The listing builds one solid part. Answer for the finished solid, in the listing's coordinates (mm). Face numbers are marked on the shaded views. A direction names the side the tool comes from. Give positions to 0.01 mm unless a question says otherwise; leave off trailing zeros. Write each loop counter-clockwise with the first axis right and the second up, starting at its lowest first coordinate (ties: lowest second). Pieces come first, ordered by that corner, then holes. Notation, with made-up numbers: (-19.5, -9.5) -> (15.5, -9.5) arc R21 cw to (15.5, 19.5) -> close; hole circle Ø8 at (-30, 19). An arc over 180 degrees is marked (long way). Use CSV: the item, a comma, the result in double quotes. Start each with the question number.
from build123d import *

# Parameters (mm, degrees)
SKETCH_1_W          = 42
SKETCH_1_H          = 15
EXTRUDE_1_DEPTH     = 5
SKETCH_2_W          = 22
SKETCH_2_H          = 25
EXTRUDE_2_DEPTH     = 9.5
CUT_EXTRUDE_1_DEPTH = 37


with BuildPart() as part:
    # 스케치1 → 보스-돌출1 (new body)
    with BuildSketch(Plane.XY):
        Rectangle(SKETCH_1_W, SKETCH_1_H)
    extrude(amount=EXTRUDE_1_DEPTH)

    # 스케치2 → 보스-돌출2 (add)
    with BuildSketch(Plane.XY.offset(5)):
        Rectangle(SKETCH_2_W, SKETCH_2_H)
    extrude(amount=EXTRUDE_2_DEPTH)

    # 스케치3 → 컷-돌출1 (cut)
    with BuildSketch(Plane(origin=(11, 0, 0), x_dir=(0, 0, -1), z_dir=(1, 0, 0))):
        Polygon((-12.28944968, 12.5), (-5.909253868, -12.5), (-14.5, -12.5), (-14.5, 12.5), align=None)
    extrude(amount=-CUT_EXTRUDE_1_DEPTH, mode=Mode.SUBTRACT)


solid = part.part
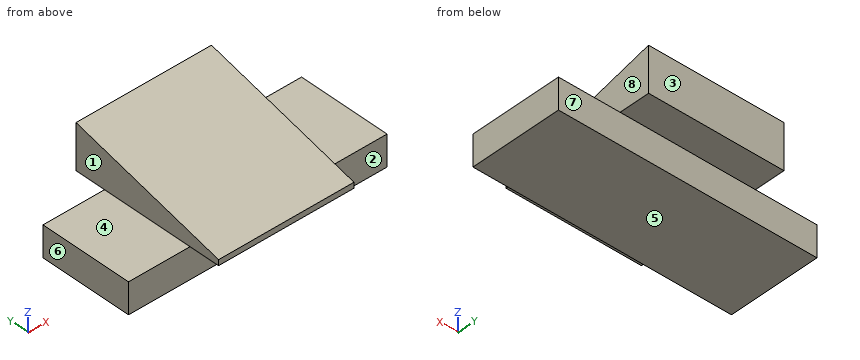
Q1. Section A-A on x = 0 is taken. Give the vertices of the cut face in (y, z).
Q2. For the marked faces 4, 5, 6, 7 and 8, determine the directions among +Z, -Z, +X, -X, +Y, -Y from which every point of the face is accessible in a straight line to the end or side of a thin tool.
Q3. Section B-B on y = -4.5 is taken. Give the vertices of the cut face in (x, z), then the cut area to 3 significant figures.
Q4. Section C-C on z = 3.5 is taken. Give the vertices of the cut face in (x, y).
Q5. Flat-ended cylindrical pins translate along their axes: pin 1 Ø2 at (x, z) = (12.5, 10.5) entering from +Y; pin 2 Ø12 at (x, y) = (16.5, -3) entering from -Z; pin 3 Ø2 at (x, z) = (12.5, 4.5) entering from -Y; pin 4 Ø8 at (x, y) = (-4, 7) entering from +Z. Find the tip coordinate at first contact, or state that the pin passes through.
Q6. Section D-D on x = 18 is taken. Give the vertices of the cut face in (y, z), then the cut area to 3 significant figures.
Q7. Straight lines are drawn through the part: L1, parallel to Y at x = 0.5, z = 4.5; L2, parallel to X at y = 1.5, z = 8.5; L3, parallel to Z at x = 14, y = -0.5. For each, find the intervals that lie inside material, in ascending order.
Q8. The mould has two halves that part along Y. Classify the marked faces 1, 2 and 3: +Y half, -Y half, draft (parallel to the pull), parting line (faces both ways), or undercut.
Output:
1,outline,"(-12.5, 5) -> (-7.5, 5) -> (-7.5, 0) -> (7.5, 0) -> (7.5, 5) -> (12.5, 5) -> (12.5, 12.29) -> (-12.5, 5.91) -> close"
2,face 4,"+Z, -X, +Y, -Y"
2,face 5,"-Z, +X, -X, +Y, -Y"
2,face 6,"+Z, -Z, -X, +Y, -Y"
2,face 7,"-Z, +X, -X, +Y"
2,face 8,"+Z, +X, +Y, -Y"
3,outline,"(-21, 0) -> (21, 0) -> (21, 5) -> (11, 5) -> (11, 7.95) -> (-11, 7.95) -> (-11, 5) -> (-21, 5) -> close"
3,area,"275 mm²"
4,outline,"(-21, -7.5) -> (21, -7.5) -> (21, 7.5) -> (-21, 7.5) -> close"
5,pin 1,"through"
5,pin 2,"z = 0"
5,pin 3,"y = -7.5"
5,pin 4,"z = 11.91"
6,outline,"(-7.5, 0) -> (7.5, 0) -> (7.5, 5) -> (-7.5, 5) -> close"
6,area,"75.0 mm²"
7,L1,"-7.5 to 7.5"
7,L2,"-11 to 11"
7,L3,"0 to 5"
8,face 1,"draft"
8,face 2,"-Y half"
8,face 3,"+Y half"
